Part model, mm, in its own coordinate system. Face numbers are marked on the shaded views. A direction names the side the tool comes from. Round coordinates to 2 decimals unless told otherwise and drop trailing zeros. Write each loop counter-clockwise with the first axis right and the second up, starting at its lowest first coordinate (ties: lowest second). Pieces come first, ordered by that corner, then holes. Notation, with made-up numbers: M -3,-1 L 13,-1 A14 ccw 13,4 Z; hole C 13,71 d6. An arc over 180 degrees is marked long. Use a Markdown table: item, result. Add a question column.
1) Two-plate mould, pull along Z, no slides. Class the marked faces 1, 2 and 3: released by +Z, released by -Z, zero draft, split by the parting line, or undercut.
2) Which spindle directions (+Z, -Z, +X, -X, +Y, -Y) get a long thin tool onto all of the face, cutting with end or side? Do the marked faces 4 and 5. Say none if no direction does.
3) Slice it at A-A on z = -26.5. Write the cut outline in (x, y).
4) Wall check: probe 1 along X at (y, z) = (3.5, -45); probe 2 along Z at (x, y) = (94.5, 13); probe 3 along Y at (x, z) = (50.5, -4.5). Give the ranges that are in metal, low to high.
5) Slice it at D-D on z = -5. Write the cut outline in (x, y).
6) Slice it at B-B on x = 59. Write the cut outline in (y, z), plus the area to 3 significant figures.
7) Slice it at C-C on y = 26. Write the cut outline in (x, z).
```python
from build123d import *

# Parameters (mm, degrees)
SKETCH1_W           = 164
SKETCH1_H           = 84
BOSS_EXTRUDE1_DEPTH = 40
SHELL1_T            = -2
SKETCH2_W           = 150
SKETCH2_H           = 70
CUT_EXTRUDE1_DEPTH  = 2


with BuildPart() as part:
    # Sketch1 → Boss-Extrude1 (new body)
    with BuildSketch(Plane(origin=(0, 0, 0), x_dir=(1, 0, 0), z_dir=(0, 1, 0))):
        with Locations((82, 42)):
            Rectangle(SKETCH1_W, SKETCH1_H)
    extrude(amount=BOSS_EXTRUDE1_DEPTH)

    # Shell1
    shell1_openings = [part.faces().sort_by_distance(p)[0] for p in [
        (82, 40, -42),
    ]]
    offset(amount=SHELL1_T, openings=shell1_openings, kind=Kind.INTERSECTION)

    # Sketch2 → Cut-Extrude1 (cut)
    with BuildSketch(Plane(origin=(0, 2, 0), x_dir=(1, 0, 0), z_dir=(0, 1, 0))):
        with Locations((82, 42)):
            Rectangle(SKETCH2_W, SKETCH2_H)
    extrude(amount=-CUT_EXTRUDE1_DEPTH, mode=Mode.SUBTRACT)


solid = part.part
```
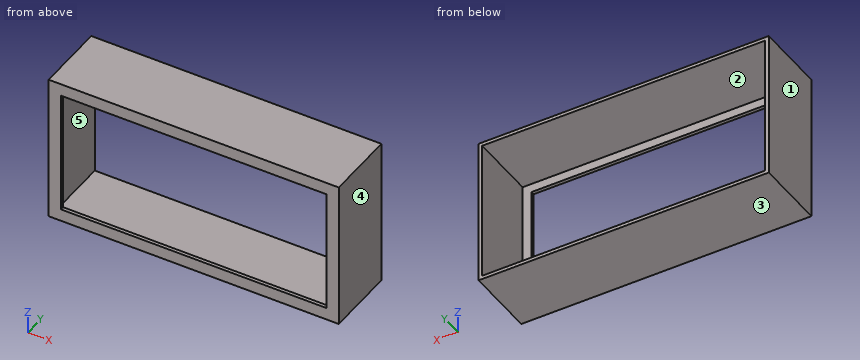
Entries:
| question | item | result |
|---|---|---|
| 1 | face 1 | zero draft |
| 1 | face 2 | undercut |
| 1 | face 3 | released by -Z |
| 2 | face 4 | +Z, -Z, +X, +Y, -Y |
| 2 | face 5 | +Y |
| 3 | outline | M 0,0 L 7,0 L 7,2 L 2,2 L 2,40 L 0,40 Z; M 157,0 L 164,0 L 164,40 L 162,40 L 162,2 L 157,2 Z |
| 4 | probe 1 | x = 0 to 2, 162 to 164 |
| 4 | probe 2 | z = -84 to -82, -2 to 0 |
| 4 | probe 3 | y = 0 to 2 |
| 5 | outline | M 0,0 L 164,0 L 164,40 L 162,40 L 162,2 L 2,2 L 2,40 L 0,40 Z |
| 6 | outline | M 0,-84 L 40,-84 L 40,-82 L 2,-82 L 2,-77 L 0,-77 Z; M 0,-7 L 2,-7 L 2,-2 L 40,-2 L 40,0 L 0,0 Z |
| 6 | area | 180 mm^2 |
| 7 | outline | M 0,-84 L 164,-84 L 164,0 L 0,0 Z; hole M 2,-82 L 162,-82 L 162,-2 L 2,-2 Z |
